from build123d import *

# Parameters (mm, degrees)
SKETCH3_R           = 1.5
CUT_EXTRUDE1_DEPTH  = 20
BOSS_EXTRUDE2_START = 36
BOSS_EXTRUDE2_DEPTH = 8
CIRPATTERN1_COUNT   = 8
SKETCH5_R           = 4.669864721
CUT_EXTRUDE2_DEPTH  = 37
CUT_EXTRUDE4_DEPTH  = 34
CUT_EXTRUDE4_DRAFT  = -0.5
BOSS_EXTRUDE3_DEPTH = 7


with BuildPart() as part:
    # Sketch2 → Revolve1 (revolve)
    with BuildSketch(Plane.XY):
        Polygon((13, 0), (13, 36), (22.5, 36), (32.5, 36), (32.5, 0), align=None)
    revolve(axis=Axis((0, 0, 0), (0, 1, 0)))

    # Sketch3 → Cut-Extrude1 (cut)
    with BuildSketch(Plane(origin=(0, 36, 0), x_dir=(1, 0, 0), z_dir=(0, 1, 0))):
        with Locations((-17.4, 0)):
            Circle(SKETCH3_R)
        with Locations((17.4, 0)):
            Circle(SKETCH3_R)
    extrude(amount=-CUT_EXTRUDE1_DEPTH, mode=Mode.SUBTRACT)

    # Sketch4 → Boss-Extrude2 (add)
    with BuildSketch(Plane(origin=(0, 0, 0), x_dir=(1, 0, 0), z_dir=(0, 1, 0)).offset(BOSS_EXTRUDE2_START)):
        with BuildLine():
            Line((0, 34.5), (-10.606601718, 45.106601718))
            ThreePointArc((-10.606601718, 45.106601718), (-14.215943039, 44.102295655), (-17.732352445, 42.809685765))
            Line((-17.732352445, 42.809685765), (-12.437211552, 30.026084807))
            ThreePointArc((-12.437211552, 30.026084807), (0, 32.5), (12.437211552, 30.026084807))
            Line((12.437211552, 30.026084807), (17.732352445, 42.809685765))
            ThreePointArc((17.732352445, 42.809685765), (14.215943039, 44.102295655), (10.606601718, 45.106601718))
            Line((10.606601718, 45.106601718), (0, 34.5))
        make_face()
    boss_extrude2 = extrude(amount=-BOSS_EXTRUDE2_DEPTH)

    # CirPattern1: Boss-Extrude2 ×8 about axis
    cirpattern1_axis = Axis((0, 0, 0), (0, 1, 0))
    for i in range(1, CIRPATTERN1_COUNT):
        add(boss_extrude2.rotate(cirpattern1_axis, i * 360 / CIRPATTERN1_COUNT))

    # Sketch5 → Cut-Extrude2 (cut, through all)
    with BuildSketch(Plane(origin=(0, 36, 0), x_dir=(1, 0, 0), z_dir=(0, 1, 0))):
        with Locations((11.791900395, 5.472758453)):
            Circle(SKETCH5_R)
    extrude(amount=-CUT_EXTRUDE2_DEPTH, mode=Mode.SUBTRACT)


with BuildPart() as cut_extrude4_tool:
    # Sketch8 → Cut-Extrude4 (with draft: the straight prism first)
    with BuildSketch(Plane.XZ):
        with BuildLine():
            Line((-19.5, 19.5), (-19.5, -19.5))
            Line((-19.5, -19.5), (-4, -19.5))
            ThreePointArc((-4, -19.5), (0, -23.5), (4, -19.5))
            Line((4, -19.5), (19.5, -19.5))
            Line((19.5, -19.5), (19.5, 19.5))
            Line((19.5, 19.5), (-19.5, 19.5))
        make_face()
    extrude(amount=-CUT_EXTRUDE4_DEPTH)
    # Cut-Extrude4: the draft: its side faces are tilted about the plane it starts from
    cut_extrude4_sides = [cut_extrude4_tool.faces().sort_by_distance(p)[0] for p in [
        (-19.5, 17, 0),
        (-11.75, 17, -19.5),
        (0, 17, -23.5),
        (11.75, 17, -19.5),
        (19.5, 17, 0),
        (0, 17, 19.5),
    ]]
    draft(cut_extrude4_sides, Plane.XZ, CUT_EXTRUDE4_DRAFT)


with BuildPart() as part_1:
    add(part.part)

    # Cut-Extrude4: cut by cut_extrude4_tool
    add(cut_extrude4_tool.part, mode=Mode.SUBTRACT)

    # Sketch9 → Boss-Extrude3 (add)
    with BuildSketch(Plane(origin=(0, 36, 0), x_dir=(1, 0, 0), z_dir=(0, 1, 0))):
        with BuildLine():
            ThreePointArc((-16.715121997, -14.30400981), (20.325349715, 8.419035512), (-21.933838447, -1.704913777))
            ThreePointArc((-21.933838447, -1.704913777), (-27.254446209, -11.289161255), (-16.715121997, -14.30400981))
        make_face()
        with BuildLine():
            ThreePointArc((-19.646781143, -3.742190633), (-25.406687144, -10.52379439), (-16.538500547, -11.246243802))
            ThreePointArc((-16.538500547, -11.246243802), (18.47759065, 7.653668647), (-19.646781143, -3.742190633))
        make_face(mode=Mode.SUBTRACT)
    extrude(amount=BOSS_EXTRUDE3_DEPTH)


solid = part_1.part
Could you check a few things on this model? Use its own coordinates, in mm. A direction names the side the tool comes from. Give positions to 0.01 mm unless a question says otherwise; leave off trailing zeros. Order: outer loops, then holes, each group sorted by start corner. A loop starts at its lowest first (then second) coordinate and runs counter-clockwise, first axis right, second up.
1. Suppose I cut it at C-C (y = 10.5). List the corners of the cut face in (x, z) for me.
2. I need wall thicknesses on L1, parallel to Z at x = 0, y = 41.75; L2, parallel to Z at x = 0, y = 34.9; L3, parallel to Y at x = 7, z = 28.5. Which ranges of each line are inside material? Lowest first, please.
3. Will these pins go through, and if not, where does the flat tip stop? P1, Ø2.5, axis at x = -28.5, y = 31.5, coming from the -Z side; P2, Ø4, axis at y = 32.5, z = -33.5, coming from the -X side; P3, Ø5, axis at x = 13, y = 19, coming from the +Z side; P4, Ø5, axis at x = -24, z = -17.5, coming from the -Y side.
4. We'd pull the mould along Z, two halves only. Please class faces 4 (the flat face through (-24.395, 32, 32)), 5 (the cylindrical face through (16.075, 35.014, -7.334)), 6 (the flat face through (32, 32, -24.395)): pulls with the +Z half, pulls with the -Z half, needs draft (parallel to the pull), parting line crosses it, or undercut.
5. For faces 1 (the flat face through (-5.2, 32.1, -39.7)), 2 (the conical face through (-0.089, 16.762, -23.353)), 3 (the flat face through (39.7, 32.1, -5.2)), which set-ups out of +Z, -Z, +X, -X, +Y, -Y let a thin tool reach every point of the face, with its end or its side?
6. Suppose I cut it at B-B (y = 21.5). List the corners of the cut face in (x, z) for me, plus the area to 3 significant figures.
7. Suppose I cut it at A-A (x = 36). List the corners of the cut face in (y, z) for me.
Solved:
1. outline: circle Ø65 at (0, 0); hole (-19.41, -19.41) - (-3.91, -19.41) arc R3.91 ccw (long way) to (3.91, -19.41) - (19.41, -19.41) - (19.41, 19.41) - (-19.41, 19.41) - close
2. L1: z = -22 to -20, 20 to 22
2. L2: z = -34.5 to -13, 13 to 34.5
2. L3: y = 0 to 36
3. P1: stops at z = -24.4
3. P2: stops at x = -24.4
3. P3: stops at z = 30.76
3. P4: stops at y = 0
4. face 4: needs draft
4. face 5: undercut
4. face 6: pulls with the -Z half
5. face 1: -Z, +Y, -Y
5. face 2: -Y
5. face 3: +X, +Y, -Y
6. outline: circle Ø65 at (0, 0); hole (-19.31, -19.31) - (-3.81, -19.31) arc R3.81 ccw (long way) to (3.81, -19.31) - (19.31, -19.31) - (19.31, 19.31) - (-19.31, 19.31) - close
6. area: 1,800 mm2
7. outline: (28, -24.4) - (36, -24.4) - (36, -1.5) - (28, -1.5) - close; (28, 1.5) - (36, 1.5) - (36, 24.4) - (28, 24.4) - close
